Geometry check sheet. Reference: the model listing, model coordinates, mm. Face numbers are marked on the shaded views. A direction names the side the tool comes from. Round coordinates to 2 decimals unless told otherwise and drop trailing zeros. Loops run counter-clockwise (first coordinate to the right, second up) from the corner with the lowest first, then second, coordinate; pieces in that order, holes last. Notation, with made-up numbers: (83, -29.75) - (138, -29.75) arc R14 cw to (138, -12.75) - close; hole circle Ø10 at (-23, 86). An arc over 180 degrees is marked (long way). Write item = value, one per line.
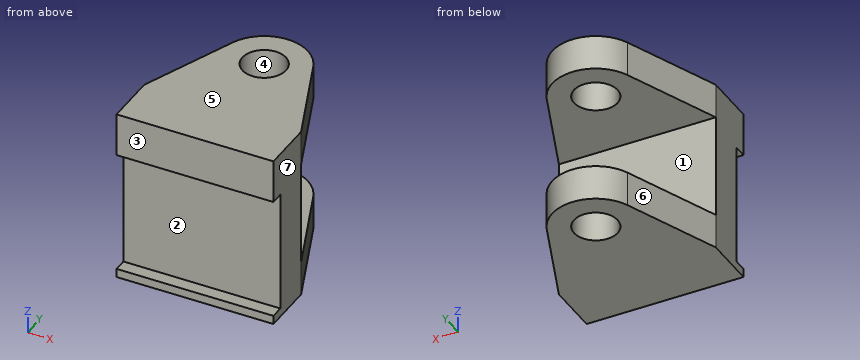
```python
from build123d import *

# Parameters (mm, degrees)
SKETCH_1_R               = 5
SKETCH_1_W               = 18
SKETCH_1_H               = 6
EXTRUDE_1_DEPTH          = 10
CUT_EXTRUDE_1_DEPTH      = 27.702059846
CUT_EXTRUDE_1_DEPTH_BACK = 27.702059846
SKETCH_2_W               = 14
SKETCH_2_H               = 3
CUT_EXTRUDE_START        = -4
CUT_EXTRUDE_2_DEPTH      = 12
CUT_EXTRUDE_3_DEPTH      = 28.748873851
CUT_EXTRUDE_3_DEPTH_BACK = 28.748873851
SKETCH_4_R               = 2.5


with BuildPart() as part:
    # 草图1 → 凸台-拉伸1 (new, symmetric)
    with BuildSketch(Plane.XY):
        with Locations((0, 12)):
            Circle(SKETCH_1_R)
        with BuildLine():
            Line((9, 3), (4.64019442, 13.862416642))
            ThreePointArc((4.64019442, 13.862416642), (4.909224587, 12.948427093), (5, 12))
            ThreePointArc((5, 12), (-0.948427093, 7.090775413), (-4.64019442, 13.862416642))
            Line((-4.64019442, 13.862416642), (-9, 3))
            Line((-9, 3), (9, 3))
        make_face()
        Rectangle(SKETCH_1_W, SKETCH_1_H)
    extrude(amount=EXTRUDE_1_DEPTH, both=True)

    # 草图2 → 切除-拉伸1 (cut, two sides: drawn at the far end of the back side and taken through both)
    with BuildSketch(Plane(origin=(9, 0, 0), x_dir=(0, 0, -1), z_dir=(1, 0, 0)).offset(-CUT_EXTRUDE_1_DEPTH_BACK)):
        with Locations((2, -3)):
            Rectangle(SKETCH_2_W, SKETCH_2_H)
    extrude(amount=CUT_EXTRUDE_1_DEPTH + CUT_EXTRUDE_1_DEPTH_BACK, mode=Mode.SUBTRACT)

    # 草图3 → 切除-拉伸2 (cut)
    with BuildSketch(Plane.XY.offset(10).offset(CUT_EXTRUDE_START)):
        with BuildLine():
            Line((-9, 3), (9, 3))
            Line((9, 3), (4.64019442, 13.862416642))
            ThreePointArc((4.64019442, 13.862416642), (0, 17), (-4.64019442, 13.862416642))
            Line((-4.64019442, 13.862416642), (-9, 3))
        make_face()
    extrude(amount=-CUT_EXTRUDE_2_DEPTH, mode=Mode.SUBTRACT)

    # 草图4 → 切除-拉伸3 (cut, two sides: drawn at the far end of the back side and taken through both)
    with BuildSketch(Plane.XY.offset(10).offset(-CUT_EXTRUDE_3_DEPTH_BACK)):
        with Locations((0, 12)):
            Circle(SKETCH_4_R)
    extrude(amount=CUT_EXTRUDE_3_DEPTH + CUT_EXTRUDE_3_DEPTH_BACK, mode=Mode.SUBTRACT)


solid = part.part
```
(1) Scan lines: L1, parallel to Y at x = 0, z = -8.25; L2, parallel to Z at x = -3.75, y = 9; L3, parallel to X at y = 16, z = 8. Record each from-to range of solid material in increasing order. Write a range as [from, to].
Answers follow:
L1 = [-1.5, 9.5], [14.5, 17]
L2 = [-10, -6], [6, 10]
L3 = [-3, 3]
(2) Section check B-B (x = 0). Enter the section's corners in (y, z).
Answers follow:
outline = (-3, -10) - (9.5, -10) - (9.5, -6) - (3, -6) - (3, 6) - (9.5, 6) - (9.5, 10) - (-3, 10) - (-3, 5) - (-1.5, 5) - (-1.5, -9) - (-3, -9) - close; (14.5, -10) - (17, -10) - (17, -6) - (14.5, -6) - close; (14.5, 6) - (17, 6) - (17, 10) - (14.5, 10) - close
(3) Section check D-D (x = -4). Enter the section's corners in (y, z).
Answers follow:
outline = (-3, -10) - (15, -10) - (15, -6) - (3, -6) - (3, 6) - (15, 6) - (15, 10) - (-3, 10) - (-3, 5) - (-1.5, 5) - (-1.5, -9) - (-3, -9) - close
(4) Mould release check, pull along X, two halves, no side actions. Record for the marked faces 4, 5, 6 and 7: pulls with the +X half, pulls with the -X half, needs draft (parallel to the pull), parting line crosses it, or undercut.
Answers follow:
face_4 = undercut
face_5 = needs draft
face_6 = pulls with the -X half
face_7 = pulls with the +X half
(5) Gauge pin test, flat ends, axial feed: pin 1 (1.5 mm diameter, centred on x = -1.5, z = -6, fed in from -Y); pin 2 (1.5 mm diameter, centred on x = 1, z = 8, fed in from +Y); pin 3 (4 mm diameter, centred on x = 0, y = 12, fed in from -Z). Record the tip position at first contact, or that the pin passes through.
Answers follow:
pin_1 = -1.5
pin_2 = 16.99
pin_3 = through
(6) Set-up check for the marked faces 1, 2 and 3: record each of +Z, -Z, +X, -X, +Y, -Y from which the full face is reachable in a straight line by a thin tool's end or side.
Answers follow:
face_1 = +X, -X, +Y
face_2 = +X, -X, -Y
face_3 = +Z, -Z, +X, -X, -Y
(7) Section check C-C (y = 8.75). Enter the section's corners in (x, z), then the cut area to 3 significant figures.
Answers follow:
outline = (-6.69, -10) - (6.69, -10) - (6.69, -6) - (-6.69, -6) - close; (-6.69, 6) - (6.69, 6) - (6.69, 10) - (-6.69, 10) - close
area = 107 mm²
(8) Section check A-A (y = 12). Enter the section's corners in (x, z), then the cut area to 3 significant figures.
Answers follow:
outline = (-5.39, -10) - (-2.5, -10) - (-2.5, -6) - (-5.39, -6) - close; (-5.39, 6) - (-2.5, 6) - (-2.5, 10) - (-5.39, 10) - close; (2.5, -10) - (5.39, -10) - (5.39, -6) - (2.5, -6) - close; (2.5, 6) - (5.39, 6) - (5.39, 10) - (2.5, 10) - close
area = 46.2 mm²
